from build123d import *

# Parameters (mm, degrees)
SKETCH_W   = 280
SKETCH_H   = 530
SKETCH_R   = 2
SKETCH_W_2 = 185
SKETCH_H_2 = 500
SKETCH_W_3 = 50
PAD_DEPTH  = 2


with BuildPart() as part:
    # Sketch → Pad (new body)
    with BuildSketch(Plane.XY):
        Rectangle(SKETCH_W, SKETCH_H)
        with Locations((-132.5, 125)):
            Circle(SKETCH_R, mode=Mode.SUBTRACT)
        with Locations((-132.5, -125)):
            Circle(SKETCH_R, mode=Mode.SUBTRACT)
        with Locations((132.5, -125)):
            Circle(SKETCH_R, mode=Mode.SUBTRACT)
        with Locations((132.5, 125)):
            Circle(SKETCH_R, mode=Mode.SUBTRACT)
        with Locations((-32.5, 0)):
            Rectangle(SKETCH_W_2, SKETCH_H_2, mode=Mode.SUBTRACT)
        with Locations((100, 0)):
            Rectangle(SKETCH_W_3, SKETCH_H_2, mode=Mode.SUBTRACT)
    extrude(amount=PAD_DEPTH)


solid = part.part
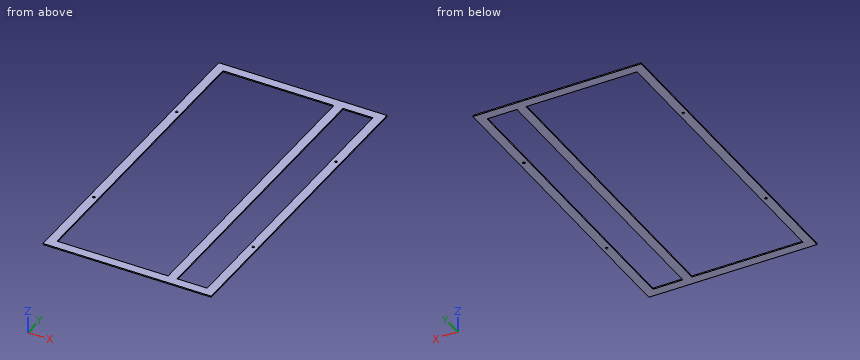
Geometry check sheet. Reference: the model listing, model coordinates, mm. Round coordinates to 2 decimals unless told otherwise and drop trailing zeros. Write each loop counter-clockwise with the first axis right and the second up, starting at its lowest first coordinate (ties: lowest second). Pieces come first, ordered by that corner, then holes. Notation, with made-up numbers: (74.5, 54) - (115.5, 54) arc R20 cw to (115.5, 61) - close; hole circle Ø9 at (29, -16). An arc over 180 degrees is marked (long way). One line per item, written item: value.
1. Depth check by flat-ended pin: pin 1 Ø5 at (x, y) = (-132.5, 125) entering from -Z. Enter the tip coordinate at first touch or a pass-through.
The answers:
pin 1: stops at z = 0
2. Cross-section at A-A on y = 34. Record the boundary of the cut face in (x, z).
The answers:
outline: (-140, 0) - (-125, 0) - (-125, 2) - (-140, 2) - close; (60, 0) - (75, 0) - (75, 2) - (60, 2) - close; (125, 0) - (140, 0) - (140, 2) - (125, 2) - close
3. Cross-section at B-B on z = 0.9. Record the boundary of the cut face in (x, y), and give its area (3 significant figures).
The answers:
outline: (-140, -265) - (140, -265) - (140, 265) - (-140, 265) - close; hole circle Ø4 at (-132.5, -125); hole circle Ø4 at (-132.5, 125); hole (-125, -250) - (60, -250) - (60, 250) - (-125, 250) - close; hole (75, -250) - (125, -250) - (125, 250) - (75, 250) - close; hole circle Ø4 at (132.5, -125); hole circle Ø4 at (132.5, 125)
area: 30,800 mm^2
4. Scan lines: L1, parallel to X at y = -118.5, z = 1.9; L2, parallel to Y at x = 132.5, z = 1.25; L3, parallel to Y at x = -93.5, z = 0.35. Record each from-to range of solid material in increasing order.
The answers:
L1: x = -140 to -125, 60 to 75, 125 to 140
L2: y = -265 to -127, -123 to 123, 127 to 265
L3: y = -265 to -250, 250 to 265
